from build123d import *

# Parameters (mm, degrees)
SKETCH1_W           = 324
SKETCH1_H           = 324
BOSS_EXTRUDE1_DEPTH = 8
SKETCH2_R           = 7.5
CUT_EXTRUDE1_DEPTH  = 8
SKETCH3_R           = 45
CUT_EXTRUDE2_DEPTH  = 10
CIRPATTERN1_COUNT   = 4
FILLET1_R           = 15


with BuildPart() as part:
    # Sketch1 → Boss-Extrude1 (new body)
    with BuildSketch(Plane.XY):
        Rectangle(SKETCH1_W, SKETCH1_H)
    extrude(amount=BOSS_EXTRUDE1_DEPTH)

    # Sketch2 → Cut-Extrude1 (cut)
    with BuildSketch(Plane.XY.offset(8)):
        with Locations((58.336309448, 58.336309448)):
            Circle(SKETCH2_R)
    cut_extrude1 = extrude(amount=-CUT_EXTRUDE1_DEPTH, mode=Mode.SUBTRACT)

    # Sketch3 → Cut-Extrude2 (cut)
    with BuildSketch(Plane.XY.offset(8)):
        Circle(SKETCH3_R)
    extrude(amount=-CUT_EXTRUDE2_DEPTH, mode=Mode.SUBTRACT)

    # CirPattern1: Cut-Extrude1 ×4 about axis
    cirpattern1_axis = Axis((0, 0, 0), (0, 0, 1))
    for i in range(1, CIRPATTERN1_COUNT):
        add(cut_extrude1.rotate(cirpattern1_axis, i * 360 / CIRPATTERN1_COUNT), mode=Mode.SUBTRACT)

    # Fillet1
    fillet1_edges = [part.edges().sort_by_distance(p)[0] for p in [
        (162, -162, 4),
        (-162, -162, 4),
        (-162, 162, 4),
        (162, 162, 4),
    ]]
    fillet(fillet1_edges, radius=FILLET1_R)


solid = part.part
Can you work these out from the model? Positions are in its coordinate system, mm. Give positions to 0.01 mm unless a question says otherwise; leave off trailing zeros. Order: outer loops, then holes, each group sorted by start corner. A loop starts at its lowest first (then second) coordinate and runs counter-clockwise, first axis right, second up. Notation, with made-up numbers: M 79,79 L 121,79 A4 ccw 121,86 Z; hole C -2,48 d2. An arc over 180 degrees is marked long. One line per question, with ' | ' between items.
Item 1: Suppose I cut it at C-C, the plane z = 4.5. Write out the boundary of the cut face in (x, y), then the cut area to 3 significant figures.
Answer block:
outline: M -162,-147 A15 ccw -147,-162 L 147,-162 A15 ccw 162,-147 L 162,147 A15 ccw 147,162 L -147,162 A15 ccw -162,147 Z; hole C -58.34,-58.34 d15; hole C -58.34,58.34 d15; hole C 0,0 d90; hole C 58.34,-58.34 d15; hole C 58.34,58.34 d15 | area: 97,700 mm2
Item 2: We'd pull the mould along X, two halves only. Please class faces 1 (the face through (-2, -162, 4)), 2 (the face through (157.49, 157.72, 4.06)), 3 (the face through (20.765, -39.923, 4.056)): released by +X, released by -X, zero draft, split by the parting line, or undercut.
Answer block:
face 1: zero draft | face 2: released by +X | face 3: undercut
Item 3: Suppose I cut it at A-A, the plane x = -36. Write out the boundary of the cut face in (y, z).
Answer block:
outline: M -162,0 L -27,0 L -27,8 L -162,8 Z; M 27,0 L 162,0 L 162,8 L 27,8 Z
Item 4: Please list where these lines run through material, in increasing order: L1, parallel to X at y = 1.5, z = 7 (3 decimals); L2, parallel to X at y = 60, z = 2.5; L3, parallel to X at y = 13, z = 2.5.
Answer block:
L1: x = -162 to -44.975, 44.975 to 162 | L2: x = -162 to -65.65, -51.02 to 51.02, 65.65 to 162 | L3: x = -162 to -43.08, 43.08 to 162
Item 5: Suppose I cut it at B-B, the plane y = 0. Write out the boundary of the cut face in (x, z), then the cut area to 3 significant figures.
Answer block:
outline: M -162,0 L -45,0 L -45,8 L -162,8 Z; M 45,0 L 162,0 L 162,8 L 45,8 Z | area: 1,870 mm2
